Design review of the part built by this model. Coordinates are the model's own, in mm. A direction names the side the tool comes from. Round coordinates to 2 decimals unless told otherwise and drop trailing zeros. Order: outer loops, then holes, each group sorted by start corner. A loop starts at its lowest first (then second) coordinate and runs counter-clockwise, first axis right, second up. Notation, with made-up numbers: M -15,48.25 L 29,48.25 A31 ccw 29,76.25 Z; hole C 11,-37.75 d2. An arc over 180 degrees is marked long. Use a Markdown table: item, result. Add a question column.
(1) Take a section at C-C (x = 0). Count the separate pieces of the cut face and the enclosed holes in it, then the cut area to 3 significant figures.
(2) The part is to be moulded in two halves that separate along Y. For faces 6 (the face through (21, -140, -106)), 7 (the face through (0, -53, 0)), 8 (the face through (8, -6, 5)), say which applies: released by +Y, released by -Y, zero draft, split by the parting line, or undercut.
(3) Take a section at B-B (z = -105). Write out the cut boundary in (x, y).
(4) Take a section at D-D (z = -149). Write out the cut boundary in (x, y), then the cut area to 3 significant figures.
(5) Machinability: for faces 1 (the face through (0, -110, -220)), 2 (the face through (-10, -124, -104)), 3 (the face through (10, -124, -104)), 4 (the face through (0, -18, -220)), 5 (the face through (0, -110, -48)), which of the approach directions +Z, -Z, +X, -X, +Y, -Y give a long, thin tool a straight path to every point of the face, cutting with its end or side? Answer none if there is none.
(6) To check wall thickness, follow probe 1 along Z at (x, y) = (10.5, -121); probe 2 along Z at (x, y) = (12, -80); probe 3 along Z at (x, y) = (2, -10.5). State the ranges of each line that lie inside material, in increasing order. Write a range as from..to.
(7) Take a section at A-A (y = -67). Write out the cut boundary in (x, z).
(8) For pin 1 (1.5 mm diameter, centred on x = -2.5, z = -223.5, fed in from +Y); pin 2 (7 mm diameter, centred on x = 26.5, z = -110.5, fed in from +Y); pin 3 (22 mm diameter, centred on x = 3.5, z = -54.5, fed in from +Y); pin 4 (9 mm diameter, centred on y = -140, z = -225, fed in from +X), all flat-tipped, find the tip position at first contact; note any pin that passes through.
```python
from build123d import *

# Parameters (mm, degrees)
BOSS_EXTRUDE1_DEPTH       = 10
SKETCH2_W                 = 65
SKETCH2_H                 = 10
BOSS_EXTRUDE2_DEPTH       = 105
SKETCH3_W                 = 42
SKETCH3_H                 = 42
BOSS_EXTRUDE3_DEPTH       = 60
CHAMFER1_SIZE             = 5
BOSS_EXTRUDE6_START       = -235
BOSS_EXTRUDE6_OUTLINE_W   = 65
BOSS_EXTRUDE6_OUTLINE_H   = 20
BOSS_EXTRUDE6_DEPTH       = 15
BOSS_EXTRUDE6_START_2     = 10
BOSS_EXTRUDE6_2_OUTLINE_W = 65
BOSS_EXTRUDE6_2_OUTLINE_H = 20
BOSS_EXTRUDE6_2_DEPTH     = 15
BOSS_EXTRUDE6_START_3     = -32.5
BOSS_EXTRUDE6_3_OUTLINE_R = 5
BOSS_EXTRUDE6_3_DEPTH     = 65
BOSS_EXTRUDE9_DEPTH       = 10
BOSS_EXTRUDE9_DEPTH_BACK  = 10
SKETCH5_R                 = 5


with BuildPart() as part:
    # Sketch1 → Boss-Extrude1 (new body)
    with BuildSketch(Plane.XY):
        with BuildLine():
            Line((32.5, -150), (32.5, 0))
            ThreePointArc((32.5, 0), (0, -32.5), (-32.5, 0))
            Line((-32.5, 0), (-32.5, -150))
            Line((-32.5, -150), (32.5, -150))
        make_face()
        with BuildLine():
            ThreePointArc((-10, 0), (0, 10), (10, 0))
            Line((10, 0), (32.5, 0))
            ThreePointArc((32.5, 0), (0, 32.5), (-32.5, 0))
            Line((-32.5, 0), (-10, 0))
        make_face()
        with BuildLine():
            Line((32.5, 0), (10, 0))
            ThreePointArc((10, 0), (0, -10), (-10, 0))
            Line((-10, 0), (-32.5, 0))
            ThreePointArc((-32.5, 0), (0, -32.5), (32.5, 0))
        make_face()
    extrude(amount=BOSS_EXTRUDE1_DEPTH)

    # Sketch2 → Boss-Extrude2 (add)
    with BuildSketch(Plane(origin=(0, 0, 0), x_dir=(-1, 0, 0), z_dir=(0, 0, -1))):
        with Locations((0, -145)):
            Rectangle(SKETCH2_W, SKETCH2_H)
    extrude(amount=BOSS_EXTRUDE2_DEPTH)

    # Mirror1: part across plane


with BuildPart() as part_1:
    add(part.part)
    add(part.part.mirror(Plane(origin=(0, 0, -105), x_dir=(1, 0, 0), z_dir=(0, 0, -1))))

    # Sketch3 → Boss-Extrude3 (add)
    with BuildSketch(Plane.XY.offset(10)):
        Rectangle(SKETCH3_W, SKETCH3_H)
    extrude(amount=BOSS_EXTRUDE3_DEPTH)

    # Chamfer1
    chamfer1_edges = [part_1.edges().sort_by_distance(p)[0] for p in [
        (-21, 21, 40),
        (-21, -21, 40),
        (21, -21, 40),
        (21, 21, 40),
    ]]
    chamfer(chamfer1_edges, length=CHAMFER1_SIZE)

    # Boss-Extrude6: read off the stored shape, not the designer's step
    # Boss-Extrude6 outline → Boss-Extrude6 (add)
    with BuildSketch(Plane.XY.offset(BOSS_EXTRUDE6_START)):
        with Locations((0, -140)):
            Rectangle(BOSS_EXTRUDE6_OUTLINE_W, BOSS_EXTRUDE6_OUTLINE_H)
        with Locations((0, -80)):
            Rectangle(BOSS_EXTRUDE6_OUTLINE_W, BOSS_EXTRUDE6_OUTLINE_H)
    extrude(amount=BOSS_EXTRUDE6_DEPTH)

    # Boss-Extrude6 2 outline → Boss-Extrude6 2 (add)
    with BuildSketch(Plane.XY.offset(BOSS_EXTRUDE6_START_2)):
        with Locations((0, -140)):
            Rectangle(BOSS_EXTRUDE6_2_OUTLINE_W, BOSS_EXTRUDE6_2_OUTLINE_H)
        with Locations((0, -80)):
            Rectangle(BOSS_EXTRUDE6_2_OUTLINE_W, BOSS_EXTRUDE6_2_OUTLINE_H)
    extrude(amount=BOSS_EXTRUDE6_2_DEPTH)

    # Boss-Extrude6 3 outline → Boss-Extrude6 3 (cut)
    with BuildSketch(Plane.YZ.offset(BOSS_EXTRUDE6_START_3)):
        with BuildLine():
            ThreePointArc((-90, 15), (-87.071067812, 22.071067812), (-80, 25))
            Line((-80, 25), (-90, 25))
            Line((-90, 25), (-90, 15))
        make_face()
        with BuildLine():
            ThreePointArc((-80, 25), (-72.928932188, 22.071067812), (-70, 15))
            Line((-70, 15), (-70, 25))
            Line((-70, 25), (-80, 25))
        make_face()
        with Locations((-80, 15)):
            Circle(BOSS_EXTRUDE6_3_OUTLINE_R)
        with BuildLine():
            ThreePointArc((-130, -225), (-132.928932188, -232.071067812), (-140, -235))
            Line((-140, -235), (-130, -235))
            Line((-130, -235), (-130, -225))
        make_face()
        with BuildLine():
            ThreePointArc((-140, -235), (-147.071067812, -232.071067812), (-150, -225))
            Line((-150, -225), (-150, -235))
            Line((-150, -235), (-140, -235))
        make_face()
        with BuildLine():
            ThreePointArc((-150, 15), (-147.071067812, 22.071067812), (-140, 25))
            Line((-140, 25), (-150, 25))
            Line((-150, 25), (-150, 15))
        make_face()
        with BuildLine():
            ThreePointArc((-140, 25), (-132.928932188, 22.071067812), (-130, 15))
            Line((-130, 15), (-130, 25))
            Line((-130, 25), (-140, 25))
        make_face()
        with Locations((-140, 15)):
            Circle(BOSS_EXTRUDE6_3_OUTLINE_R)
        with BuildLine():
            ThreePointArc((-70, -225), (-72.928932188, -232.071067812), (-80, -235))
            Line((-80, -235), (-70, -235))
            Line((-70, -235), (-70, -225))
        make_face()
        with BuildLine():
            ThreePointArc((-80, -235), (-87.071067812, -232.071067812), (-90, -225))
            Line((-90, -225), (-90, -235))
            Line((-90, -235), (-80, -235))
        make_face()
        with Locations((-80, -225)):
            Circle(BOSS_EXTRUDE6_3_OUTLINE_R)
        with Locations((-140, -225)):
            Circle(BOSS_EXTRUDE6_3_OUTLINE_R)
    extrude(amount=BOSS_EXTRUDE6_3_DEPTH, mode=Mode.SUBTRACT)

    # Sketch5 → Boss-Extrude9 (add, two sides: drawn at the far end of the back side and taken through both)
    with BuildSketch(Plane(origin=(0, 0, 0), x_dir=(0, 0, -1), z_dir=(1, 0, 0)).offset(-BOSS_EXTRUDE9_DEPTH_BACK)):
        with BuildLine():
            Line((95, -110), (0, -110))
            Line((0, -110), (0, -140))
            Line((0, -140), (210, -140))
            Line((210, -140), (210, -110))
            Line((210, -110), (115, -110))
            ThreePointArc((115, -110), (105, -100), (95, -110))
        make_face()
        with Locations((105, -110)):
            Circle(SKETCH5_R, mode=Mode.SUBTRACT)
    extrude(amount=BOSS_EXTRUDE9_DEPTH + BOSS_EXTRUDE9_DEPTH_BACK)


solid = part_1.part
```
Verdict:
| question | item | result |
|---|---|---|
| 1 | separate pieces | 2 |
| 1 | enclosed holes | 5 |
| 1 | area | 15,000 mm^2 |
| 2 | face 6 | released by +Y |
| 2 | face 7 | zero draft |
| 2 | face 8 | undercut |
| 3 | outline | M -32.5,-150 L 32.5,-150 L 32.5,-140 L 10,-140 L 10,-115 L -10,-115 L -10,-140 L -32.5,-140 Z; M -10,-105 L 10,-105 L 10,-100 L -10,-100 Z |
| 4 | outline | M -32.5,-150 L 32.5,-150 L 32.5,-140 L 10,-140 L 10,-110 L -10,-110 L -10,-140 L -32.5,-140 Z |
| 4 | area | 1,250 mm^2 |
| 5 | face 1 | -Z, +X, -X |
| 5 | face 2 | -X, +Y |
| 5 | face 3 | +X, +Y |
| 5 | face 4 | -Z, +X, -X, +Y |
| 5 | face 5 | +X, -X, +Y |
| 6 | probe 1 | z = -220..-210, 0..10 |
| 6 | probe 2 | z = -235..-230, -220..-210, 0..10, 20..25 |
| 6 | probe 3 | z = -220..-210, 0..70 |
| 7 | outline | M -32.5,-220 L 32.5,-220 L 32.5,-210 L -32.5,-210 Z; M -32.5,0 L 32.5,0 L 32.5,10 L -32.5,10 Z |
| 8 | pin 1 | stops at y = -70 |
| 8 | pin 2 | stops at y = -140 |
| 8 | pin 3 | stops at y = -110 |
| 8 | pin 4 | passes through |
